Design review of the part shown in the three views and the two pictorial views. Dimensions are in mm from the part's minimum x, y and z. A direction names the side the tool comes from. Coordinates: 2 decimals unless noted, no trailing zeros. Order: outer loops, then holes, each group sorted by start corner. A loop starts at its lowest first (then second) coordinate and runs counter-clockwise, first axis right, second up. Notation, with made-up numbers: (-32.75, 70) -> (26.25, 70) arc R17 ccw to (26.25, 101) -> close; hole circle Ø8 at (-7, 52.5). An arc over 180 degrees is marked (long way). Answer as a JSON object with one key per item and string values. Group by question number.
1) Add section B-B, the plane y = 9. Write out the cut boundary in (x, z) (1 decimal).
2) Add section A-A, the plane y = 7. Write out the cut boundary in (x, z) (1 decimal).
3) Draft analysis for pull direction Y (two halves, no side actions). For the marked faces 3, 4 and 5, state which applies: +Y half, -Y half, draft (parallel to the pull), parting line (faces both ways), or undercut.
4) Wall thickness on L1, parallel to Y at x = 2.75, z = 4.25 (1 decimal); L2, parallel to X at y = 6.5, z = 13.5; L3, parallel to X at y = 5.5, z = 8.5: over which ranges is each line inside the solid? List them lowest first.
5) For pin 1 (6 mm diameter, centred on x = 6, y = 6.5, fed in from -Z); pin 2 (1 mm diameter, centred on x = 5, y = 5.5, fed in from +Z); pin 3 (1 mm diameter, centred on x = 9.5, y = 3.5, fed in from +Z) (1 decimal), all flat-tipped, find the tip position at first contact; note any pin that passes through.
6) Machinability: for the marked faces 1 and 2, which of the approach directions +Z, -Z, +X, -X, +Y, -Y give a long, thin tool a straight path to every point of the face, cutting with its end or side? Answer none if there is none.
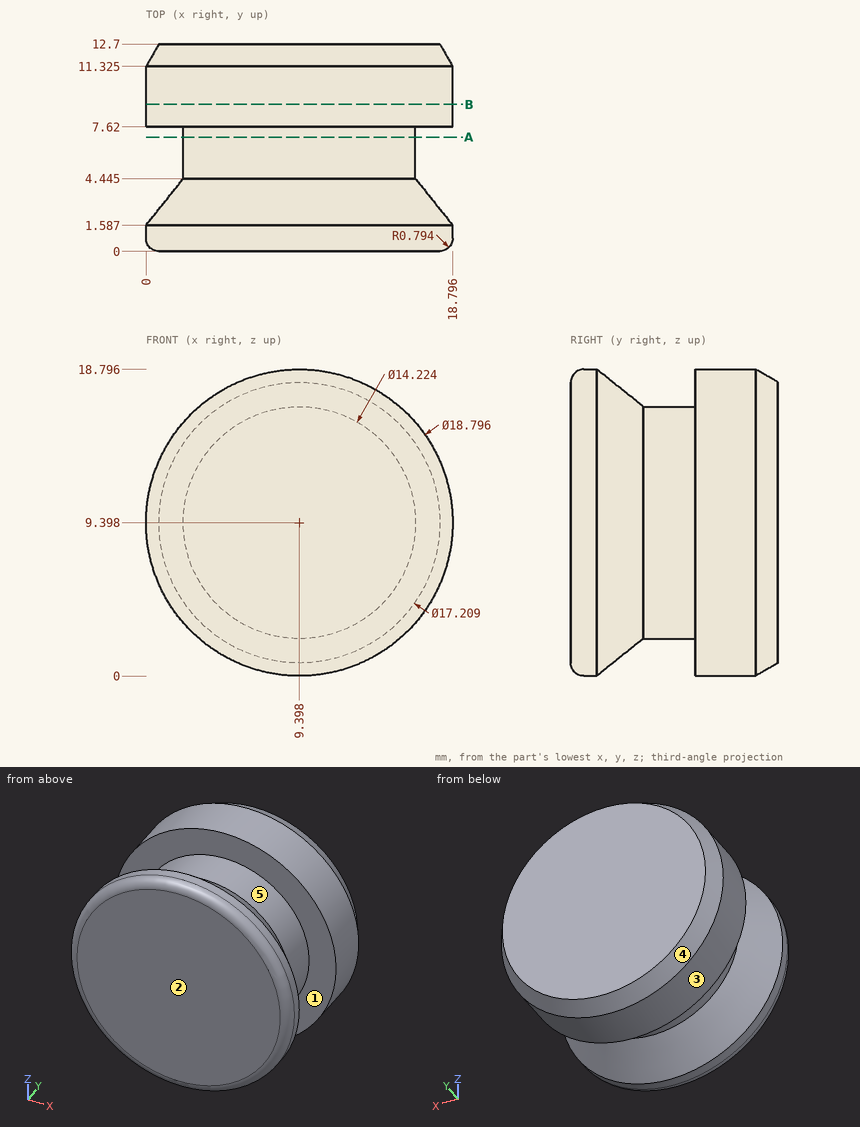
Output values:
{
 "1": {"outline": "circle Ø18.8 at (9.4, 9.4)"},
 "2": {"outline": "circle Ø14.2 at (9.4, 9.4)"},
 "3": {"face 3": "draft", "face 4": "+Y half", "face 5": "undercut"},
 "4": {"L1": "y = 0 to 2.8, 7.6 to 12.7", "L2": "x = 3.59 to 15.21", "L3": "x = 2.34 to 16.45"},
 "5": {"pin 1": "stops at z = 0.02", "pin 2": "stops at z = 15.35", "pin 3": "stops at z = 17.7"},
 "6": {"face 1": "none", "face 2": "+Z, -Z, +X, -X, -Y"}
}
